Design review of the part built by this model. Coordinates are the model's own, in mm. A direction names the side the tool comes from. Give positions to 0.01 mm unless a question says otherwise; leave off trailing zeros. Loops run counter-clockwise (first coordinate to the right, second up) from the corner with the lowest first, then second, coordinate; pieces in that order, holes last. Notation, with made-up numbers: (78, -2.5) -> (109, -2.5) arc R14 cw to (109, 5.5) -> close; hole circle Ø4 at (-9.75, 36). An arc over 180 degrees is marked (long way). Answer as CSV lines item,"result".
from build123d import *

# Parameters (mm, degrees)
SKETCH1_R              = 13
SKETCH1_R_2            = 9
BOSS_EXTRUDE1_DEPTH    = 5
SKETCH2_R              = 14
SKETCH2_R_2            = 10
BOSS_EXTRUDE2_DEPTH    = 7
CUT_EXTRUDE1_DEPTH     = 7
BOSS_EXTRUDE3_DEPTH    = 5
FILLET1_R              = 2
FILLET2_R              = 0.5
CUT_EXTRUDE2_DEPTH     = 9
BOSS_EXTRUDE4_DEPTH    = 7
FILLET3_R              = 2
FILLET4_R              = 0.5
BOSS_EXTRUDE5_START    = -18
BOSS_EXTRUDE5_DEPTH    = 18
BOSS_EXTRUDE6_START    = -18
BOSS_EXTRUDE6_DEPTH    = 18
SKETCH7_W              = 6
SKETCH7_H              = 18
BOSS_EXTRUDE7_DEPTH    = 28
FILLET5_R              = 1
CUT_EXTRUDE3_START     = -6
CUT_EXTRUDE3_OUTLINE_R = 1.1
CUT_EXTRUDE3_DEPTH     = 6
FILLET7_R              = 2


# Read off the part's stored shape, not the designer's step: Boss-Extrude6, Cut-Extrude3
# Some blends are built 0.0001 mm under size
with BuildPart() as part:
    # Sketch1 → Boss-Extrude1 (new body)
    with BuildSketch(Plane(origin=(0, 0, 0), x_dir=(1, 0, 0), z_dir=(0, 1, 0))):
        with Locations(Location((0, 0, 0), (0, 0, 270))):
            Circle(SKETCH1_R)
        with Locations(Location((0, 0, 0), (0, 0, 270))):
            Circle(SKETCH1_R_2, mode=Mode.SUBTRACT)
    extrude(amount=BOSS_EXTRUDE1_DEPTH)

    # Sketch3 → Cut-Extrude1 (cut)
    with BuildSketch(Plane.XZ):
        with BuildLine():
            ThreePointArc((12.369316877, 4), (0, 13), (-12.369316877, 4))
            Line((-12.369316877, 4), (-8.062257748, 4))
            ThreePointArc((-8.062257748, 4), (0, 9), (8.062257748, 4))
            Line((8.062257748, 4), (12.369316877, 4))
        make_face()
    extrude(amount=-CUT_EXTRUDE1_DEPTH, mode=Mode.SUBTRACT)

    # Sketch3<3> → Boss-Extrude3 (add)
    with BuildSketch(Plane.XZ):
        with BuildLine():
            Line((-7.215434845, 4), (-8.062257748, 4))
            ThreePointArc((-8.062257748, 4), (-8.477795251, 3.02109048), (-8.774964387, 2))
            Line((-8.774964387, 2), (-8.003905297, 2))
            ThreePointArc((-8.003905297, 2), (-7.675094696, 3.025792692), (-7.215434845, 4))
        make_face()
        with BuildLine():
            ThreePointArc((8.774964387, 2), (8.477795251, 3.02109048), (8.062257748, 4))
            Line((8.062257748, 4), (7.215434845, 4))
            ThreePointArc((7.215434845, 4), (7.675094696, 3.025792692), (8.003905297, 2))
            Line((8.003905297, 2), (8.774964387, 2))
        make_face()
    extrude(amount=-BOSS_EXTRUDE3_DEPTH)

    # Fillet1
    # the kernel refuses this fillet: 2 mm, written as the material it takes off along each edge
    with BuildSketch(Plane(origin=(8.003905297, -2.925457541, 2), x_dir=(-0.3106184744402921, 0, 0.9505346723483502), z_dir=(0, 1, 0))) as fillet1_piece_1:
        with BuildLine():
            CenterArc((1.312023382, 1.994963987), FILLET1_R, 219.12562277, 46.807536055)
            Line((-0.239505198, 0.7329184), (-0.27053577, 0.707677488))
            ThreePointArc((-0.27053577, 0.707677488), (-0.157773986, 0.354034461), (-0.038021387, -0.012424739))
            Line((-0.038021387, -0.012424739), (0.002836807, -0.03989928))
            ThreePointArc((0.002836807, -0.03989928), (0.585091508, -0.019226448), (1.167346209, -0.03989928))
            Line((1.167346209, -0.03989928), (1.170183016, 0))
        make_face()
    extrude(amount=10.850915082, mode=Mode.SUBTRACT)
    with BuildSketch(Plane(origin=(-8.003905297, -2.925457541, 2), x_dir=(-1, 0, 0), z_dir=(0, 1, 0))) as fillet1_piece_2:
        with BuildLine():
            CenterArc((1.488743739, 1.866796386), FILLET1_R, 202.16334775, 46.807536055)
            Line((-0.363480463, 1.11229953), (-0.400524947, 1.097209593))
            ThreePointArc((-0.400524947, 1.097209593), (-0.200015637, 0.550177675), (-0.038806814, -0.00969697))
            Line((-0.038806814, -0.00969697), (0, -0.04))
            ThreePointArc((0, -0.04), (0.385529545, -0.04), (0.756705398, -0.037335928))
            Line((0.756705398, -0.037335928), (0.771059091, 0))
        make_face()
    extrude(amount=10.850915082, mode=Mode.SUBTRACT)

    # Fillet2
    fillet2_edges = [part.edges().sort_by_distance(p)[0] for p in [
        (-12.369316877, 2.5, 4),
        (12.369316877, 2.5, 4),
        (-7.215434845, 2.5, 4),
        (7.215434845, 2.5, 4),
    ]]
    fillet(fillet2_edges, radius=FILLET2_R)



with BuildPart() as body_2:
    # Sketch2 → Boss-Extrude2 (new body)
    with BuildSketch(Plane(origin=(0, 11, 0), x_dir=(1, 0, 0), z_dir=(0, 1, 0))):
        with Locations(Location((0, 0, 0), (0, 0, 270))):
            Circle(SKETCH2_R)
        with Locations(Location((0, 0, 0), (0, 0, 270))):
            Circle(SKETCH2_R_2, mode=Mode.SUBTRACT)
    extrude(amount=BOSS_EXTRUDE2_DEPTH)

    # Sketch4 → Cut-Extrude2 (cut)
    with BuildSketch(Plane.XZ.offset(-11)):
        with BuildLine():
            ThreePointArc((13.076696831, 5), (0, 14), (-13.076696831, 5))
            Line((-13.076696831, 5), (-8.660254038, 5))
            ThreePointArc((-8.660254038, 5), (0, 10), (8.660254038, 5))
            Line((8.660254038, 5), (13.076696831, 5))
        make_face()
    extrude(amount=-CUT_EXTRUDE2_DEPTH, mode=Mode.SUBTRACT)

    # Sketch4<3> → Boss-Extrude4 (add)
    with BuildSketch(Plane.XZ.offset(-11)):
        with BuildLine():
            Line((-7.782191208, 5), (-8.660254038, 5))
            ThreePointArc((-8.660254038, 5), (-9.154604257, 4.02408013), (-9.539392014, 3))
            Line((-9.539392014, 3), (-8.75, 3))
            ThreePointArc((-8.75, 3), (-8.326363944, 4.029164115), (-7.782191208, 5))
        make_face()
        with BuildLine():
            ThreePointArc((9.539392014, 3), (9.154604257, 4.02408013), (8.660254038, 5))
            Line((8.660254038, 5), (7.782191208, 5))
            ThreePointArc((7.782191208, 5), (8.326363944, 4.029164115), (8.75, 3))
            Line((8.75, 3), (9.539392014, 3))
        make_face()
    extrude(amount=-BOSS_EXTRUDE4_DEPTH)

    # Fillet3
    # the kernel refuses this fillet: 2 mm, written as the material it takes off along each edge
    with BuildSketch(Plane(origin=(-8.75, 8.186857883, 3), x_dir=(-1, 0, 0), z_dir=(0, 1, 0))) as fillet3_piece_1:
        with BuildLine():
            CenterArc((1.370115418, 1.913833934), FILLET3_R, 205.898945897, 47.221442291)
            Line((-0.429016212, 1.040263457), (-0.464998845, 1.022792048))
            ThreePointArc((-0.464998845, 1.022792048), (-0.235653724, 0.511411041), (-0.037837838, -0.012972973))
            Line((-0.037837838, -0.012972973), (0, -0.04))
            ThreePointArc((0, -0.04), (0.394696007, -0.04), (0.777777546, -0.038276679))
            Line((0.777777546, -0.038276679), (0.789392014, 0))
        make_face()
    extrude(amount=12.626284233, mode=Mode.SUBTRACT)
    with BuildSketch(Plane(origin=(8.75, 8.186857883, 3), x_dir=(-0.3812606993131178, 0, 0.9244675652283711), z_dir=(0, 1, 0))) as fillet3_piece_2:
        with BuildLine():
            CenterArc((1.246906235, 1.996296928), FILLET3_R, 219.291406968, 47.221442291)
            Line((-0.300964151, 0.729767313), (-0.331921559, 0.704436721))
            ThreePointArc((-0.331921559, 0.704436721), (-0.187460778, 0.349633229), (-0.036978703, -0.015250428))
            Line((-0.036978703, -0.015250428), (0.002432988, -0.039925939))
            ThreePointArc((0.002432988, -0.039925939), (0.562628423, -0.022873294), (1.122823859, -0.039925939))
            Line((1.122823859, -0.039925939), (1.125256847, 0))
        make_face()
    extrude(amount=12.626284233, mode=Mode.SUBTRACT)

    # Fillet4
    fillet4_edges = [body_2.edges().sort_by_distance(p)[0] for p in [
        (-13.076696831, 14.5, 5),
        (13.076696831, 14.5, 5),
        (-7.782191208, 14.5, 5),
        (7.782191208, 14.5, 5),
    ]]
    fillet(fillet4_edges, radius=FILLET4_R)


with BuildPart() as part_1:
    add(part.part)

    add(body_2.part)  # Boss-Extrude5 merges body 2
    # Sketch5 → Boss-Extrude5 (add)
    with BuildSketch(Plane(origin=(0, 18, 0), x_dir=(1, 0, 0), z_dir=(0, 1, 0)).offset(BOSS_EXTRUDE5_START)):
        with BuildLine():
            ThreePointArc((0, 14), (4.788282007, 13.155696691), (8.999026536, 10.724622204))
            Line((8.999026536, 10.724622204), (10.284601755, 12.25671109))
            ThreePointArc((10.284601755, 12.25671109), (0, 16), (-10.284601755, 12.25671109))
            Line((-10.284601755, 12.25671109), (-8.999026536, 10.724622204))
            ThreePointArc((-8.999026536, 10.724622204), (-4.788282007, 13.155696691), (0, 14))
        make_face()
        with BuildLine():
            ThreePointArc((0, 13), (4.446261863, 12.21600407), (8.356238926, 9.958577761))
            Line((8.356238926, 9.958577761), (8.999026536, 10.724622204))
            ThreePointArc((8.999026536, 10.724622204), (4.788282007, 13.155696691), (0, 14))
            Line((0, 14), (0, 13))
        make_face()
        with BuildLine():
            Line((-8.999026536, 10.724622204), (-8.356238926, 9.958577761))
            ThreePointArc((-8.356238926, 9.958577761), (-4.446261863, 12.21600407), (0, 13))
            Line((0, 13), (0, 14))
            ThreePointArc((0, 14), (-4.788282007, 13.155696691), (-8.999026536, 10.724622204))
        make_face()
    extrude(amount=BOSS_EXTRUDE5_DEPTH)

    # Boss-Extrude6 outline → Boss-Extrude6 (add)
    with BuildSketch(Plane(origin=(0, 18, 0), x_dir=(1, 0, 0), z_dir=(0, 1, 0)).offset(BOSS_EXTRUDE6_START)):
        with BuildLine():
            ThreePointArc((-3, 15.716233646), (0, 16), (3, 15.716233646))
            Line((3, 15.716233646), (3, 17.5))
            Line((3, 17.5), (-3, 17.5))
            Line((-3, 17.5), (-3, 15.716233646))
        make_face()
    extrude(amount=BOSS_EXTRUDE6_DEPTH)

    # Sketch7 → Boss-Extrude7 (add)
    with BuildSketch(Plane(origin=(0, 0, -17.5), x_dir=(-1, 0, 0), z_dir=(0, 0, -1))):
        with Locations((0, 9)):
            Rectangle(SKETCH7_W, SKETCH7_H)
    extrude(amount=BOSS_EXTRUDE7_DEPTH)

    # Fillet5
    fillet5_edges = [part_1.edges().sort_by_distance(p)[0] for p in [
        (-8.356238926, 2.5, -9.958577761),
        (-8.999026536, 14.5, -10.724622204),
        (8.356238926, 2.5, -9.958577761),
        (8.999026536, 14.5, -10.724622204),
        (10.284601755, 9, -12.25671109),
        (-10.284601755, 9, -12.25671109),
    ]]
    fillet(fillet5_edges, radius=FILLET5_R - 0.0001)  # a hair under: the kernel refuses the full size

    # Cut-Extrude3 outline → Cut-Extrude3 (cut)
    with BuildSketch(Plane.ZY.offset(3).offset(CUT_EXTRUDE3_START)):
        with BuildLine():
            ThreePointArc((-16.032782087, 0), (-30.438112209, 1.0880478), (-44.526972297, 4.282011691))
            Line((-44.526972297, 4.282011691), (-40.332962383, 18))
            Line((-40.332962383, 18), (-45.5, 18))
            Line((-45.5, 18), (-45.5, 0))
            Line((-45.5, 0), (-16.032782087, 0))
        make_face()
        with Locations((-38.338138622, 12.915422706)):
            Circle(CUT_EXTRUDE3_OUTLINE_R)
        with BuildLine():
            Line((-32.284081469, 13.580062224), (-33.04731745, 9.65355349))
            ThreePointArc((-33.04731745, 9.65355349), (-24.421849449, 8.406791821), (-15.716233646, 8.000139171))
            Line((-15.716233646, 8.000139171), (-15.716233646, 12.000145644))
            ThreePointArc((-15.716233646, 12.000145644), (-24.038466281, 12.388378225), (-32.284081469, 13.580062224))
        make_face()
    extrude(amount=CUT_EXTRUDE3_DEPTH, mode=Mode.SUBTRACT)

    # Fillet7
    fillet7_edges = [part_1.edges().sort_by_distance(p)[0] for p in [
        (0, 12.000145644, -15.716233646),
        (0, 8.000139171, -15.716233646),
        (0, 9.65355349, -33.04731745),
        (0, 13.580062224, -32.284081469),
        (0, 18, -40.332962383),
        (0, 4.282011691, -44.526972297),
    ]]
    fillet(fillet7_edges, radius=FILLET7_R - 0.0001)  # a hair under: the kernel refuses the full size


solid = part_1.part
Q1. To check wall thickness, follow probe 1 along X at (y, z) = (16.25, 0); probe 2 along X at (y, z) = (3.9, 0); probe 3 along X at (y, z) = (1.25, -24). State the ranges of each line that lie inside material, in increasing order. Write a range as from..to.
Filled sheet:
probe 1,"x = -14..-10, 10..14"
probe 2,"x = -13..-9, 9..13"
probe 3,"x = -3..3"
Q2. For faces 1 (the cylindrical face through (-0.042, 8.606, -16.301)), 2 (the cylindrical face through (8.1, 2.46, 2.43)), 3 (the cylindrical face through (0, 14, -10)), list the 3-axis set-ups (+Z, -Z, +X, -X, +Y, -Y) from which the entire face can be reached by the end or side of a thin tool; tool diameter is ignored.
Filled sheet:
face 1,"+X, -X"
face 2,"+Y, -Y"
face 3,"+Y"
Q3. We need section B-B, the plane z = -22.5. State the section outline as (x, y) points, and give its area (3 significant figures).
Filled sheet:
outline,"(-3, 0.22) -> (3, 0.22) -> (3, 8.24) -> (-3, 8.24) -> close; (-3, 12.26) -> (3, 12.26) -> (3, 18) -> (-3, 18) -> close"
area,"82.6 mm^2"
Q4. We need section A-A, the plane z = 0. State the section outline as (x, y) points.
Filled sheet:
outline,"(-14, 11) -> (-10, 11) -> (-10, 18) -> (-14, 18) -> close; (-13, 0) -> (-9, 0) -> (-9, 5) -> (-13, 5) -> close; (9, 0) -> (13, 0) -> (13, 5) -> (9, 5) -> close; (10, 11) -> (14, 11) -> (14, 18) -> (10, 18) -> close"
Q5. Clearance check with flat-ended pins moving along their axes: pin 1 Ø5 at (x, y) = (-1, 14.5) entering from -Z; pin 2 Ø8 at (y, z) = (15.5, -33.5) entering from -X; pin 3 Ø2.5 at (y, z) = (12.92, -38.34) entering from +X; pin 4 Ø9 at (x, z) = (5.5, -4.5) entering from -Y. State where each tip first meets the part, or that it passes through.
Filled sheet:
pin 1,"stops at z = -42.17"
pin 2,"stops at x = -3"
pin 3,"stops at x = 3"
pin 4,"stops at y = 0"
Q6. The part is to be moulded in two halves that separate along Z. For faces 4 (the flat face through (0, 0, -10)), 5 (the cylindrical face through (0.042, 8.416, -24.513)), 6 (the cylindrical face through (-0.042, 17.618, -40.028)), say which applies: pulls with the +Z half, pulls with the -Z half, needs draft (parallel to the pull), parting line crosses it, or undercut.
Filled sheet:
face 4,"needs draft"
face 5,"undercut"
face 6,"pulls with the -Z half"
Q7. We need section C-C, the plane y = 10.5. State the section outline as (x, z) points, and give its area (3 significant figures).
Filled sheet:
outline,"(-9.62, -11.47) arc R1 ccw to (-9.44, -12.92) arc R16 ccw to (-3, -15.72) -> (-3, -15.77) -> (3, -15.77) -> (3, -15.72) arc R16 ccw to (9.44, -12.92) arc R1 ccw to (9.62, -11.47) -> (8.36, -9.96) arc R13 cw to (-8.36, -9.96) -> close; (-3, -42.63) -> (3, -42.63) -> (3, -32.55) -> (-3, -32.55) -> close"
area,"120 mm^2"
